from build123d import *

# Parameters (mm, degrees)
F1_DEPTH = 38.1
F2_W     = 79.502
F2_H     = 79.502
F2_W_2   = 67.31
F2_H_2   = 67.31
F3_DEPTH = 30.48
F4_DEPTH = 20.32
F6_DEPTH = 67.31
F7_R     = 2.032


with BuildPart() as f1:
    # F0 (on Front) → F1 (new body)
    with BuildSketch(Plane.XZ):
        with BuildLine():
            Line((-85.598, 0), (-2.032, 0))
            ThreePointArc((-2.032, 0), (-0.5951590206, 0.5951590206), (0, 2.032))
            Line((0, 2.032), (0, 85.598))
            ThreePointArc((0, 85.598), (-0.5951590206, 87.0348409794), (-2.032, 87.63))
            Line((-2.032, 87.63), (-85.598, 87.63))
            ThreePointArc((-85.598, 87.63), (-87.0348409794, 87.0348409794), (-87.63, 85.598))
            Line((-87.63, 85.598), (-87.63, 2.032))
            ThreePointArc((-87.63, 2.032), (-87.0348409794, 0.5951590206), (-85.598, 0))
        make_face()
    extrude(amount=F1_DEPTH)

    # F2 (on face) → F3 (cut)
    with BuildSketch(Plane(origin=(0, 0, 0), x_dir=(-1, 0, 0), z_dir=(0, 1, 0))):
        with Locations((43.815, 43.815)):
            Rectangle(F2_W, F2_H)
        with Locations((43.815, 43.815)):
            Rectangle(F2_W_2, F2_H_2, mode=Mode.SUBTRACT)
    extrude(amount=-F3_DEPTH, mode=Mode.SUBTRACT)

    # F4 (cut): a face of the model
    f4_faces = [f1.faces().sort_by_distance(p)[0] for p in [
        (-43.815, 0, 1.2392753447),
    ]]
    extrude(f4_faces, amount=-F4_DEPTH, mode=Mode.SUBTRACT)

    # F5 (on face) → F6 (cut, through all)
    with BuildSketch(Plane.XY.offset(77.47)):
        with BuildLine():
            Line((-16.658075929, 0), (-70.971924071, 0))
            ThreePointArc((-70.971924071, 0), (-43.815, -21.3715089252), (-16.658075929, 0))
        make_face()
    extrude(amount=-F6_DEPTH, mode=Mode.SUBTRACT)

    # F7
    f7_edges = [f1.edges().sort_by_distance(p)[0] for p in [
        (-43.815, -38.1, 0),
        (-0.595159, -38.1, 0.595159),
        (0, -38.1, 43.815),
        (-0.595159, -38.1, 87.034841),
        (-43.815, -38.1, 87.63),
        (-87.034841, -38.1, 87.034841),
        (-87.63, -38.1, 43.815),
        (-87.034841, -38.1, 0.595159),
    ]]
    fillet(f7_edges, radius=F7_R)


solid = f1.part
Read the model definition and answer for the solid it produces. Units are mm, in the model's axes. A direction names the side the tool comes from. Round coordinates to 2 decimals unless told otherwise and drop trailing zeros. Write each loop counter-clockwise with the first axis right and the second up, starting at its lowest first coordinate (ties: lowest second). Pieces come first, ordered by that corner, then holes. Notation, with made-up numbers: (-6.5, -6) - (25.5, -6) arc R37 ccw to (25.5, 30) - close; hole circle Ø7 at (47.25, 84.5). An arc over 180 degrees is marked (long way). One line per question, with ' | ' between items. Start each with the question number.
1. Section D-D (x = -74) is taken. Determine the outline of the cut face in (y, z).
2. Section C-C (y = -18) is taken. Determine the outline of the cut face in (x, z).
3. For faces 5 (the face through (-43, -28, 87.63)), 6 (the face through (-10.16, -15, 43)), determine the directions among +Z, -Z, +X, -X, +Y, -Y from which every point of the face is accessible in a straight line to the end or side of a thin tool.
4. Section A-A (y = -23.5) is taken. Determine the outline of the cut face in (x, z).
5. Find the intervals of material crossed by probe 1 along Z at (x, y) = (-61.5, -23); probe 2 along X at (y, z) = (-28, 44.5); probe 3 along X at (y, z) = (-22, 7.5), in increasing order. Write a range as [from, to].
6. For a pull along Z with two mould halves and no side action, classify faces 1 (the face through (-44.4, -37.49, 87.05)), 2 (the face through (0, -28, 43)), 3 (the face through (-43, -25, 83.566)), 4 (the face through (-43.23, -37.49, 0.58)) as +Z half, -Z half, draft (parallel to the pull), parting line (faces both ways), or undercut.
7. Each of these flat-tipped pins is pushed along its axis until it touches: pin 1 (10 mm diameter, centred on y = -8, z = 33, fed in from -X); pin 2 (24 mm diameter, centred on x = -41.5, z = 45.5, fed in from +Y). Where does it stop, or does it pass through?
8. Section B-B (z = 52) is taken. Determine the outline of the cut face in (x, y) (1 decimal), and give its area (3 significant figures).
Filled in:
1) outline: (-38.1, 2.03) arc R2.03 ccw to (-36.07, 0) - (-20.32, 0) - (-20.32, 4.06) - (-30.48, 4.06) - (-30.48, 10.16) - (0, 10.16) - (0, 77.47) - (-30.48, 77.47) - (-30.48, 83.57) - (-20.32, 83.57) - (-20.32, 87.63) - (-36.07, 87.63) arc R2.03 ccw to (-38.1, 85.6) - close
2) outline: (-77.47, 10.16) - (-57.12, 10.16) - (-57.12, 77.47) - (-77.47, 77.47) - close; (-30.51, 10.16) - (-10.16, 10.16) - (-10.16, 77.47) - (-30.51, 77.47) - close
3) face 5: +Z, +X, -X, +Y, -Y | face 6: +Y
4) outline: (-87.63, 2.03) arc R2.03 ccw to (-85.6, 0) - (-2.03, 0) arc R2.03 ccw to (0, 2.03) - (0, 85.6) arc R2.03 ccw to (-2.03, 87.63) - (-85.6, 87.63) arc R2.03 ccw to (-87.63, 85.6) - close; (-77.47, 10.16) - (-10.16, 10.16) - (-10.16, 77.47) - (-77.47, 77.47) - close; hole (-83.57, 4.06) - (-4.06, 4.06) - (-4.06, 83.57) - (-83.57, 83.57) - close
5) probe 1: [0, 4.06], [10.16, 77.47], [83.57, 87.63] | probe 2: [-87.63, -83.57], [-77.47, -10.16], [-4.06, 0] | probe 3: [-87.63, -83.57], [-4.06, 0]
6) face 1: +Z half | face 2: draft | face 3: undercut | face 4: -Z half
7) pin 1: x = -77.47 | pin 2: y = -17.43
8) outline: (-87.6, -36.1) arc R2 ccw to (-85.6, -38.1) - (-2, -38.1) arc R2 ccw to (0, -36.1) - (0, -20.3) - (-4.1, -20.3) - (-4.1, -30.5) - (-10.2, -30.5) - (-10.2, 0) - (-16.7, 0) arc R27.9 cw to (-71, 0) - (-77.5, 0) - (-77.5, -30.5) - (-83.6, -30.5) - (-83.6, -20.3) - (-87.6, -20.3) - close | area: 1,940 mm²
